```python
from build123d import *

# Parameters (mm, degrees)
F1_DEPTH    = 38
F2_W        = 36
F2_H        = 6
F2_R        = 2.8
F3_DEPTH    = 1
F4_DEPTH    = 4
F5_T1_DEPTH = 38.571682988


# Not quite as in the source:
# - a fillet or chamfer that OpenCascade refuses, or shapes differently, is made with other operations: its cross-section is extruded or revolved along the edge and cut away or added


with BuildPart() as f1:
    # F0 (on Top) → F1 (new body)
    with BuildSketch(Plane.XY):
        with BuildLine():
            ThreePointArc((0, 2), (0.5857864376, 0.5857864376), (2, 0))
            Line((2, 0), (38, 0))
            ThreePointArc((38, 0), (39.4142135624, 0.5857864376), (40, 2))
            Line((40, 2), (40, 23))
            ThreePointArc((40, 23), (40.5857864376, 24.4142135624), (42, 25))
            Line((42, 25), (45, 25))
            ThreePointArc((45, 25), (46.4142135624, 25.5857864376), (47, 27))
            Line((47, 27), (47, 30))
            ThreePointArc((47, 30), (46.4142135624, 31.4142135624), (45, 32))
            Line((45, 32), (40, 32))
            Line((40, 32), (37, 32))
            ThreePointArc((37, 32), (35.5857864376, 31.4142135624), (35, 30))
            Line((35, 30), (35, 9))
            ThreePointArc((35, 9), (33.5355339059, 5.4644660941), (30, 4))
            Line((30, 4), (2, 4))
            ThreePointArc((2, 4), (0.5857864376, 3.4142135624), (0, 2))
        make_face()
    extrude(amount=F1_DEPTH)

    # F2 (on face) → F3 (join)
    with BuildSketch(Plane.XZ):
        with Locations((20, 9)):
            Rectangle(F2_W, F2_H)
        with Locations((17, 9)):
            Circle(F2_R, mode=Mode.SUBTRACT)
    extrude(amount=F3_DEPTH)

    # F4 (cut): a face of the model
    f4_faces = [f1.faces().sort_by_distance(p)[0] for p in [
        (17, 0, 9),
    ]]
    extrude(f4_faces, amount=-F4_DEPTH, mode=Mode.SUBTRACT)

    # F5: chamfer of 0.5 on 1 edges, made by hand

    # F5_s2 → F5_t1 (cut)
    with BuildSketch(Plane.YZ.offset(0.714158506)):
        Polygon((-0.5, 6), (-1, 6.5), (-1, 6), align=None)
    extrude(amount=F5_T1_DEPTH, mode=Mode.SUBTRACT)


solid = f1.part
```
Source: CAD feature listing. Evaluate the final solid. Frame: model axes, mm. A direction names the side the tool comes from. Coordinates: 2 decimals unless noted, no trailing zeros. Loops run counter-clockwise (first coordinate to the right, second up) from the corner with the lowest first, then second, coordinate; pieces in that order, holes last. Notation, with made-up numbers: (45.25, -39.5) -> (99.25, -39.5) arc R24 ccw to (99.25, -12.5) -> close; hole circle Ø2 at (71.5, -38.5). An arc over 180 degrees is marked (long way). One line per item, written item: value. Start each with the question number.
Q1. Section query A-A, the plane x = 17. Return the cut outline in (y, z).
Q2. Section query C-C, the plane z = 30. Return the cut outline in (x, y).
Q3. Section query B-B, the plane z = 9. Return the cut outline in (x, y), and give its area (3 significant figures).
Q4. Set-up query: faces 5 (the face through (20, 0, 25)), 6 (the face through (20, 0, 3)), 7 (the face through (43, 25, 19)). Return all of +Z, -Z, +X, -X, +Y, -Y with unobstructed straight access to the full face (end or side cutting, diameter ignored); none if empty.
Q5. Contact query for flat-ended pins moving along their axis: P1, Ø12, axis at x = 31.5, y = 28, coming from the +Z side; P2, Ø6.5, axis at y = 12.5, z = 13, coming from the +X side; P3, Ø22.5, axis at x = 20, z = 24, coming from the +Y side; P4, Ø10.5, axis at y = 16.5, z = 13, coming from the -X side. Output: stop coordinate, or through.
Q6. Line query: line 1 along X through (y, z) = (2.05, 9); line 2 along Z through (x, y) = (17, 1.5); line 3 along X through (y, z) = (28.5, 6.5). Output: solid intervals per line, ascending.
Q7. Mould query, pull axis Z, two halves, no side actions, for faces 1 (the face through (36, 11, 38)), 2 (the face through (14.2, 1.5, 9.1)), 3 (the face through (36, 11, 0)), 4 (the face through (20, -1, 10)). Classes: pulls with the +Z half, pulls with the -Z half, needs draft (parallel to the pull), parting line crosses it, or undercut.
Results:
1. outline: (-1, 11.8) -> (4, 11.8) -> (4, 38) -> (0, 38) -> (0, 12) -> (-1, 12) -> close; (-0.7, 6.2) -> (-0.5, 6) -> (0, 6) -> (0, 0) -> (4, 0) -> (4, 6.2) -> close
2. outline: (2, 0) -> (38, 0) arc R2 ccw to (40, 2) -> (40, 23) arc R2 cw to (42, 25) -> (45, 25) arc R2 ccw to (47, 27) -> (47, 30) arc R2 ccw to (45, 32) -> (37, 32) arc R2 ccw to (35, 30) -> (35, 9) arc R5 cw to (30, 4) -> (2, 4) arc R2 ccw to start
3. outline: (2, -1) -> (14.2, -1) -> (14.2, 4) -> (2, 4) arc R2 ccw to (2, 0) -> close; (19.8, -1) -> (38, -1) -> (38, 0) arc R2 ccw to (40, 2) -> (40, 23) arc R2 cw to (42, 25) -> (45, 25) arc R2 ccw to (47, 27) -> (47, 30) arc R2 ccw to (45, 32) -> (37, 32) arc R2 ccw to (35, 30) -> (35, 9) arc R5 cw to (30, 4) -> (19.8, 4) -> close
3. area: 358 mm^2
4. face 5: +Z, +X, -X, -Y
4. face 6: -Z, +X, -X, -Y
4. face 7: +Z, -Z, +X, -Y
5. P1: z = 38
5. P2: x = 40
5. P3: y = 4.16
5. P4: x = 35
6. line 1: 0 to 14.2, 19.8 to 40
6. line 2: 0 to 6.2, 11.8 to 38
6. line 3: 35 to 47
7. face 1: pulls with the +Z half
7. face 2: undercut
7. face 3: pulls with the -Z half
7. face 4: needs draft
